The listing builds one solid part. Answer for the finished solid, in the listing's coordinates (mm). A direction names the side the tool comes from. Give positions to 0.01 mm unless a question says otherwise; leave off trailing zeros. Order: outer loops, then holes, each group sorted by start corner. A loop starts at its lowest first (then second) coordinate and runs counter-clockwise, first axis right, second up. Notation, with made-up numbers: (83, 64.25) - (109, 64.25) arc R7 cw to (109, 75.25) - close; hole circle Ø5 at (48.5, 29). An arc over 180 degrees is marked (long way). Answer as CSV lines item,"result". Start each with the question number.
1. Which of the six approach directions +Z, -Z, +X, -X, +Y, -Y give full straight-line access (tool end or side, diameter ignored) to faces 1 (the flat face through (-9, 2, 15)), 2 (the flat face through (-9, 2, -15)), 3 (the flat face through (-11.5, 0, 0.1))?
2. Determine the mould class of faces 4 (the flat face through (-8, 1, 20.5)), 5 (the flat face through (-13, 1, 0)), 6 (the cylindrical face through (12, 4, -5)), 7 (the cylindrical face through (-2.38, 4.44, -10.74)) for opening direction Z: +Z half, -Z half, draft (parallel to the pull), parting line (faces both ways), or undercut.
3. Section C-C on y = 7 is taken. Give the vertices of the cut face in (x, z), and give its area (3 significant figures).
4. Section A-A on x = 0 is taken. Give the vertices of the cut face in (y, z).
5. Section D-D on x = -8 is taken. Give the vertices of the cut face in (y, z), and give its area (3 significant figures).
6. Consider line 1 along X through (y, z) = (6, 0); line 2 along Z through (x, y) = (-8, 1). Determine where each line is inside the solid, lowest interval first. Write a range as [from, to].
7. Flat-ended cylindrical pins translate along their axes: pin 1 (3.5 mm diameter, centred on x = -8, z = 17.49, fed in from +Y); pin 2 (8 mm diameter, centred on x = 6, z = 13.5, fed in from -Y); pin 3 (1 mm diameter, centred on y = 1, z = -17, fed in from +X); pin 4 (3 mm diameter, centred on x = 7.5, y = 4.5, fed in from +Z). Find the tip coordinate at first contact, or state that the pin passes through.
Autodesk Inventor part; units mm, degrees
ref_plane "YZ Plane" through (0, 0, 0) normal (1, 0, 0) x (0, 1, 0)
ref_plane "XZ Plane" through (0, 0, 0) normal (0, 1, 0) x (-1, 0, 0)
ref_plane "XY Plane" through (0, 0, 0) normal (0, 0, 1) x (1, 0, 0)
sketch "Sketch3" plane through (0, 0, 0) normal (0, 1, 0) x (-1, 0, 0)
  line L0 (3, -20.5) -> (3, -14.5)
  line L1 (13, 20.5) -> (3, 20.5)
  line L2 (3, -20.5) -> (3, 20.5)
  line L3 (3, 20.5) -> (13, 20.5)
  line L4 (13, 20.5) -> (13, -20.5)
  line L5 (13, -20.5) -> (3, -20.5)
  line L6 (0, 0) -> (3, 0)
  line L7 (13, 14.5) -> (3, 14.5)
  line L8 (3, -14.5) -> (13, -14.5)
  line L9 (3, -14.5) -> (13, -14.5)
  line L10 (3, 14.5) -> (13, 14.5)
  circle A0 centre (8, -17.508) radius 1.425
  circle A1 centre (8, -17.508) radius 1.425
  circle A2 centre (8, 17.4854) radius 1.425
  circle A3 centre (8, 17.4854) radius 1.425
  point P0 (3, 20.5)
  dimension "d15" = 41
  dimension "d16" = 10
  dimension "d17" = 0
  dimension "d18" = 6
extrude "Extrusion1" add sketch "Sketch3" along normal blind 2
sketch "Sketch5" plane through (0, 0, 0) normal (0, -1, 0) x (1, 0, 0)
  line L0 (-3, 20.5) -> (-3, 14.5)
  line L1 (-13, -20.5) -> (-3, -20.5)
  line L2 (-3, 20.5) -> (-3, -20.5)
  line L3 (-3, -20.5) -> (-13, -20.5)
  line L4 (-13, -20.5) -> (-13, 20.5)
  line L5 (-13, 20.5) -> (-3, 20.5)
  line L6 (0, 0) -> (-3, 0)
  line L7 (-13, -14.5) -> (-3, -14.5)
  line L8 (-3, 14.5) -> (-13, 14.5)
  line L9 (-3, 14.5) -> (-13, 14.5)
  line L10 (-3, -14.5) -> (-13, -14.5)
  circle A0 centre (-8, 17.508) radius 1.425
  circle A1 centre (-8, 17.508) radius 1.425
  circle A2 centre (-8, -17.4854) radius 1.425
  circle A3 centre (-8, -17.4854) radius 1.425
  circle A4 centre (0, 0) radius 11
  circle A5 centre (0, 0) radius 13
  point P0 (3, 20.5)
  point P1 (3, -14.5)
  point P2 (-3, 12.6491)
  point P3 (-3, 10.583)
  point P4 (-3, -10.583)
  point P5 (-3, -12.6491)
  dimension "d27" = 41
  dimension "d28" = 10
  dimension "d29" = 0
  dimension "d30" = 6
  dimension "d31" = 22
  dimension "d32" = 26
extrude "Extrusion2" add sketch "Sketch5" against normal blind 9 contours A5 L2 A4 | L2 A4 A5
sketch "Sketch6" plane through (0, 9, 0) normal (0, 1, 0) x (1, 0, 0)
  circle A0 centre (0, 0) radius 11
extrude "Extrusion3" cut sketch "Sketch6" against normal through all
properties part number "Ball_Bearing_Holder"
Checks:
1,face 1,"+Z, -X, +Y"
1,face 2,"-Z, -X, +Y"
1,face 3,"+Z, -Z, +X, -X, -Y"
2,face 4,"+Z half"
2,face 5,"draft"
2,face 6,"parting line"
2,face 7,"undercut"
3,outline,"circle Ø26 at (0, 0); hole circle Ø22 at (0, 0)"
3,area,"151 mm²"
4,outline,"(0, -13) - (9, -13) - (9, -11) - (0, -11) - close; (0, 11) - (9, 11) - (9, 13) - (0, 13) - close"
5,outline,"(0, -20.5) - (2, -20.5) - (2, -18.93) - (0, -18.93) - close; (0, -16.08) - (2, -16.08) - (2, -10.25) - (9, -10.25) - (9, -7.55) - (0, -7.55) - close; (0, 7.55) - (9, 7.55) - (9, 10.25) - (2, 10.25) - (2, 16.06) - (0, 16.06) - close; (0, 18.91) - (2, 18.91) - (2, 20.5) - (0, 20.5) - close"
5,area,"78.2 mm²"
6,line 1,"x = [-13, -11], [11, 13]"
6,line 2,"z = [-20.5, -18.93], [-16.08, -7.55], [7.55, 16.06], [18.91, 20.5]"
7,pin 1,"stops at y = 2"
7,pin 2,"stops at y = 0"
7,pin 3,"stops at x = -3"
7,pin 4,"stops at z = 11.53"
